Check sheet for the drawn part. Datum: minimum x, y, z corner. Units: mm. Give positions to 0.01 mm unless a question says otherwise; leave off trailing zeros. Order: outer loops, then holes, each group sorted by start corner. A loop starts at its lowest first (then second) coordinate and runs counter-clockwise, first axis right, second up. Notation, with made-up numbers: (56, 43) - (74, 43) arc R24 cw to (74, 76) - close; hole circle Ø8 at (-33, 37). An arc over 180 degrees is marked (long way). Answer as a JSON object with one key per item and string values. Group by question number.
(1) Thickness scan on line 1 (Z direction, x = 434.5, y = 11.5); line 2 (X direction, y = 11.75, z = 86); line 3 (Z direction, x = 172, y = 11.5). Record the ranges inside material, lowest first.
(2) Section check B-B (x = 167). Record the boundary of the cut face in (y, z), then the cut area to 3 significant figures.
(3) Section check A-A (z = 426.5). Record the boundary of the cut face in (x, y), then the cut area to 3 significant figures.
(4) Section check C-C (y = 3). Count the separate pieces of the cut face and the enclosed holes in it, then the cut area to 3 significant figures.
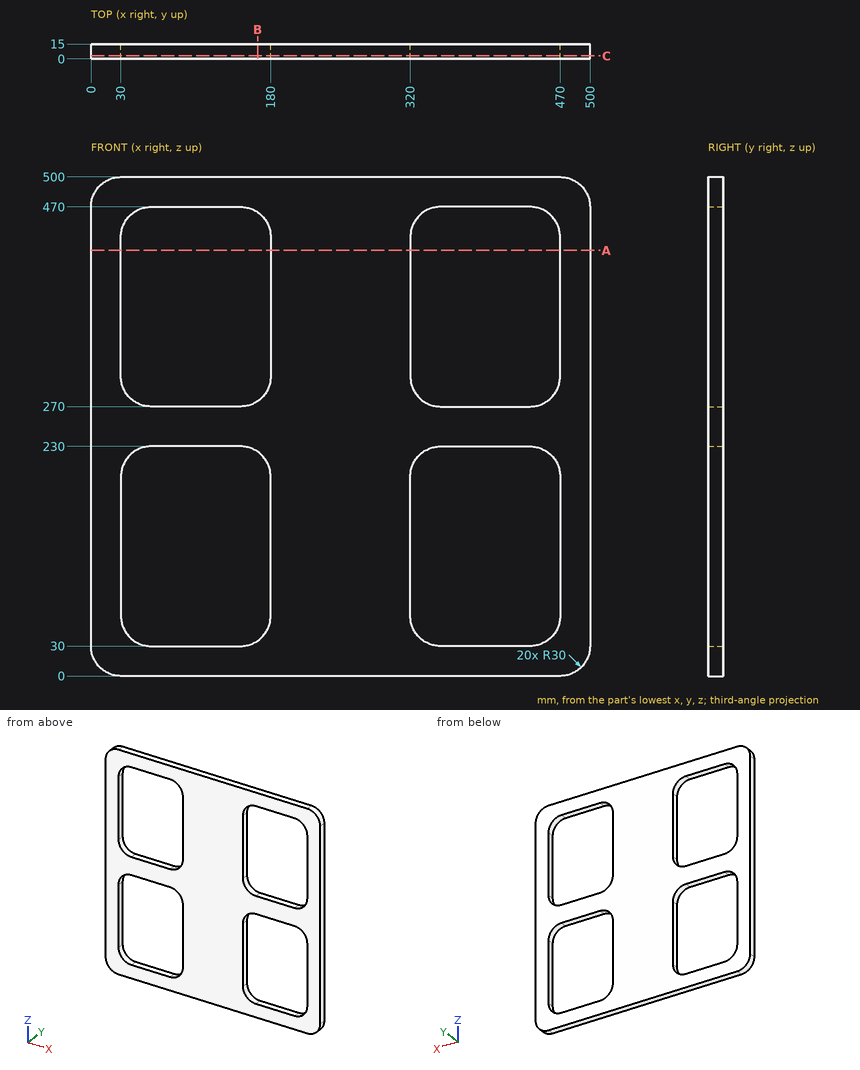
Solutions:
{
 "1": {"line 1": "z = 0 to 30, 230 to 270, 470 to 500", "line 2": "x = 0 to 30, 180 to 320, 470 to 500", "line 3": "z = 0 to 39.6, 220.4 to 279.6, 460.4 to 500"},
 "2": {"outline": "(0, 0) - (15, 0) - (15, 35.28) - (0, 35.28) - close; (0, 224.72) - (15, 224.72) - (15, 275.28) - (0, 275.28) - close; (0, 464.72) - (15, 464.72) - (15, 500) - (0, 500) - close", "area": "1,820 mm2"},
 "3": {"outline": "(0, 0) - (30, 0) - (30, 15) - (0, 15) - close; (180, 0) - (320, 0) - (320, 15) - (180, 15) - close; (470, 0) - (500, 0) - (500, 15) - (470, 15) - close", "area": "3,000 mm2"},
 "4": {"separate pieces": "1", "enclosed holes": "4", "area": "132,000 mm2"}
}
